```python
from build123d import *

# Parameters (mm, degrees)
SKETCH2_R           = 2.5
BOSS_EXTRUDE1_DEPTH = 10
CHAMFER1_SIZE       = 0.5
CUT_EXTRUDE1_DEPTH  = 2.3
SKETCH8_R           = 1.782050808
CUT_EXTRUDE2_DEPTH  = 1
CUT_EXTRUDE2_TAPER  = 45


with BuildPart() as part:
    # Sketch2 → Boss-Extrude1 (new body)
    with BuildSketch(Plane(origin=(0, 0, 0), x_dir=(0, 0, -1), z_dir=(1, 0, 0))):
        Circle(SKETCH2_R)
    extrude(amount=-BOSS_EXTRUDE1_DEPTH)

    # Chamfer1
    chamfer1_edges = [part.edges().sort_by_distance(p)[0] for p in [
        (0, 0, 2.5),
    ]]
    chamfer(chamfer1_edges, length=CHAMFER1_SIZE)

    # Sketch6 → Revolve1 (revolve)
    with BuildSketch(Plane.XY):
        with BuildLine():
            Line((-11.5, 0), (-11.5, 4.161437828))
            ThreePointArc((-11.5, 4.161437828), (-10.75, 4.5), (-10, 4.161437828))
            Line((-10, 4.161437828), (-10, 0))
            Line((-10, 0), (-11.5, 0))
        make_face()
    revolve(axis=Axis((-10, 0, 0), (-1, 0, 0)))

    # Sketch7 → Cut-Extrude1 (cut)
    with BuildSketch(Plane.ZY.offset(11.5)):
        Polygon((0, 1.732050808), (-1.5, 0.866025404), (-1.5, -0.866025404), (0, -1.732050808), (1.5, -0.866025404), (1.5, 0.866025404), align=None)
    extrude(amount=-CUT_EXTRUDE1_DEPTH, mode=Mode.SUBTRACT)

    # Sketch8 → Cut-Extrude2 (cut)
    with BuildSketch(Plane.ZY.offset(11.5)):
        Circle(SKETCH8_R)
    extrude(amount=-CUT_EXTRUDE2_DEPTH, taper=CUT_EXTRUDE2_TAPER, mode=Mode.SUBTRACT)


solid = part.part
```
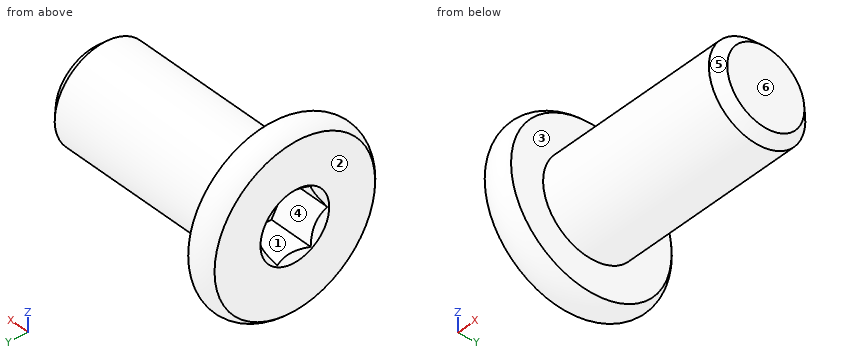
Part model, mm, in its own coordinate system. Face numbers are marked on the shaded views. A direction names the side the tool comes from. Round coordinates to 2 decimals unless told otherwise and drop trailing zeros. Loops run counter-clockwise (first coordinate to the right, second up) from the corner with the lowest first, then second, coordinate; pieces in that order, holes last. Notation, with made-up numbers: (-19.5, 89.5) -> (18.5, 89.5) arc R36 ccw to (18.5, 126.5) -> close; hole circle Ø8 at (35, -27). An arc over 180 degrees is marked (long way). Use CSV: the item, a comma, the result in double quotes. Start each with the question number.
1) Wall check: L1, parallel to X at y = -2.25, z = 2.5; L2, parallel to Z at x = -4.75, y = 2; L3, parallel to Z at x = -1, y = 1.5. Give the ranges that are in metal, low to high. Write a range as [from, to].
2) Which spindle directions (+Z, -Z, +X, -X, +Y, -Y) get a long thin tool onto all of the face, cutting with end or side? Do the marked faces 1, 2 and 3. Say none if no direction does.
3) Cut at A-A, the plane x = -5.5. Write the cut outline in (y, z), plus the area to 3 significant figures.
4) Pull direction Y, two halves, no side cores. Call the marked faces 4, 5 and 6: +Y half, -Y half, draft (parallel to the pull), parting line (faces both ways), or undercut.
5) Drop flat-ended pins along their axis: P1, Ø5, axis at x = -1, z = -3.5, coming from the -Y side; P2, Ø2.5, axis at y = 0, z = 0, coming from the -X side; P3, Ø1.5, axis at x = -8.5, y = -3, coming from the +Z side. Give the stop position or say it passes through.
Determined:
1,L1,"x = [-11.5, -10]"
1,L2,"z = [-1.5, 1.5]"
1,L3,"z = [-2, 2]"
2,face 1,"-X"
2,face 2,"+Z, -Z, -X, +Y, -Y"
2,face 3,"+X"
3,outline,"circle Ø5 at (0, 0)"
3,area,"19.6 mm2"
4,face 4,"undercut"
4,face 5,"parting line"
4,face 6,"draft"
5,P1,"stops at y = -2.29"
5,P2,"stops at x = -9.2"
5,P3,"stops at z = 1.09"
